```python
from build123d import *

# Parameters (mm, degrees)
BOSS_EXTRUDE2_DEPTH = 13.56
SKETCH5_R           = 5.7
CUT_EXTRUDE1_DEPTH  = 1002.036692109


with BuildPart() as part:
    # Sketch4 → Boss-Extrude2 (new body)
    with BuildSketch(Plane.XY):
        Polygon((-225.81606276, 70.095146264), (974.18393724, 70.095146264), (574.18393724, -229.904853736), (174.18393724, -229.904853736), align=None)
        Polygon((574.18393724, -216.344853736), (936.447387254, 55.352733774), (-188.079512773, 55.352733774), (174.18393724, -216.344853736), align=None, mode=Mode.SUBTRACT)
    extrude(amount=BOSS_EXTRUDE2_DEPTH)

    # Sketch5 → Cut-Extrude1 (cut, through all)
    with BuildSketch(Plane.XY.offset(13.56)):
        with Locations((945.339868666, 62.77782)):
            Circle(SKETCH5_R)
        with Locations((-200.789433704, 62.77782)):
            Circle(SKETCH5_R)
        with Locations((176.91916089, -223.073008716)):
            Circle(SKETCH5_R)
        with Locations((566.674885297, -223.073008716)):
            Circle(SKETCH5_R)
    extrude(amount=-CUT_EXTRUDE1_DEPTH, mode=Mode.SUBTRACT)


solid = part.part
```
Input: part model. Units: mm. Frame: model coordinates. A direction names the side the tool comes from. Give positions to 0.01 mm unless a question says otherwise; leave off trailing zeros. Loops run counter-clockwise (first coordinate to the right, second up) from the corner with the lowest first, then second, coordinate; pieces in that order, holes last.
1) Line query: L1, parallel to Y at x = 235.5, z = 10; L2, parallel to X at y = -158, z = 11; L3, parallel to X at y = 7.5, z = 3.75. Output: solid intervals per line, ascending.
A:
L1: y = -229.9 to -216.34, 55.35 to 70.1
L2: x = 78.31 to 96.39, 651.98 to 670.06
L3: x = -142.36 to -124.28, 872.64 to 890.72
2) Contact query for flat-ended pins moving along their axis: pin 1 (3 mm diameter, centred on y = -114.5, z = 10, fed in from +X); pin 2 (5 mm diameter, centred on y = -20.5, z = 9, fed in from -X); pin 3 (15 mm diameter, centred on x = -200.79, y = 62.78, fed in from -Z); pin 4 (5 mm diameter, centred on y = 25.5, z = 10.5, fed in from +X). Output: stop coordinate, or through.
A:
pin 1: stops at x = 730.06
pin 2: stops at x = -108.36
pin 3: stops at z = 0
pin 4: stops at x = 918.06
3) Section query A-A on x = 140.5. Return the cut outline in (y, z).
A:
outline: (-204.64, 0) - (-191.08, 0) - (-191.08, 13.56) - (-204.64, 13.56) - close; (55.35, 0) - (70.1, 0) - (70.1, 13.56) - (55.35, 13.56) - close
4) Reachability of faces 1 (the flat face through (-23.02, -82, 6.69)), 2 (the flat face through (-9.484, -78.594, 6.685)) from +Z, -Z, +X, -X, +Y, -Y: full face, straight path, thin tool, end or side. Return the list, or none.
A:
face 1: +Z, -Z, -X, -Y
face 2: +Z, -Z
5) Section query B-B on y = -62. Return the cut outline in (x, z), and give its area (3 significant figures).
A:
outline: (-49.69, 0) - (-31.61, 0) - (-31.61, 13.56) - (-49.69, 13.56) - close; (779.98, 0) - (798.06, 0) - (798.06, 13.56) - (779.98, 13.56) - close
area: 490 mm2
6) Section query C-C on z = 7. Return the cut outline in (x, y), and give its area (3 significant figures).
A:
outline: (-225.82, 70.1) - (174.18, -229.9) - (574.18, -229.9) - (974.18, 70.1) - close; hole circle Ø11.4 at (-200.79, 62.78); hole (-188.08, 55.35) - (174.18, -216.34) - (574.18, -216.34) - (936.45, 55.35) - close; hole circle Ø11.4 at (176.92, -223.07); hole circle Ø11.4 at (566.67, -223.07); hole circle Ø11.4 at (945.34, 62.78)
area: 32,500 mm2
7) Mould query, pull axis Y, two halves, no side actions, for faces 3 (the flat face through (377, 65, 0)), 4 (the flat face through (752.78, -82.4, 6.69)), 5 (the flat face through (776.984, -77.805, 6.685)). Classes: released by +Y, released by -Y, zero draft, split by the parting line, or undercut.
A:
face 3: zero draft
face 4: undercut
face 5: released by -Y
